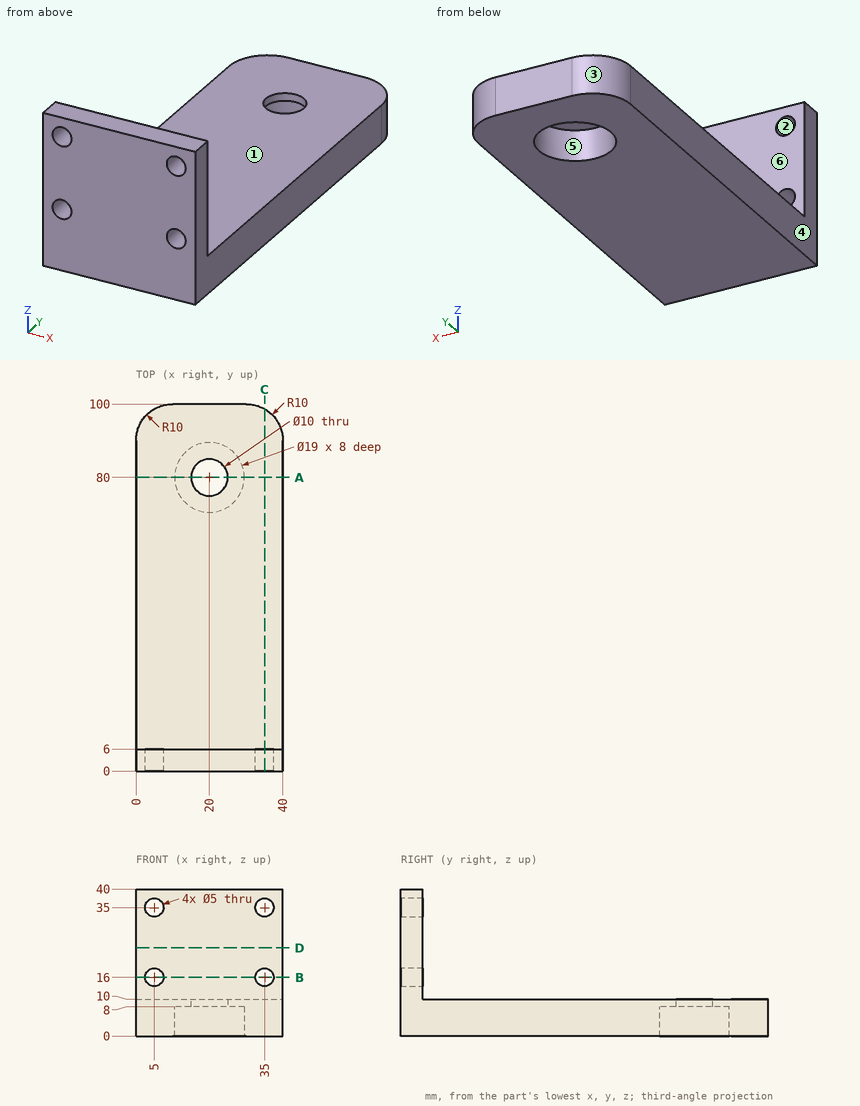
Answer from the drawing. Dimensions are ordinates in mm from the lowest x, y and z of the part. A direction names the side the tool comes from. Round coordinates to 2 decimals unless told otherwise and drop trailing zeros. Loops run counter-clockwise (first coordinate to the right, second up) from the corner with the lowest first, then second, coordinate; pieces in that order, holes last. Notation, with made-up numbers: (-5.75, -4) - (0.25, -4) arc R10 cw to (0.25, 9) - close; hole circle Ø2 at (19.5, 5.5). An arc over 180 degrees is marked (long way). Return JSON: item names as keys, results as strings. Group by question number.
1. Which of the six approach directions +Z, -Z, +X, -X, +Y, -Y give full straight-line access (tool end or side, diameter ignored) to the marked faces 4, 5 and 6?
2. The part is cut by section C-C on x = 35. Determine the outline of the cut face in (y, z).
3. The part is cut by section B-B on z = 16. Determine the outline of the cut face in (x, y), then the cut area to 3 significant figures.
4. The part is cut by section A-A on y = 80. Determine the outline of the cut face in (x, z), then the cut area to 3 significant figures.
5. The part is cut by section D-D on z = 24. Determine the outline of the cut face in (x, y).
6. Consider probe 1 along X at (y, z) = (4.05, 35); probe 2 along Y at (x, z) = (20, 9.55); probe 3 along Z at (x, y) = (11.5, 9.5). Determine where each line is inside the solid, lowest interval first.
7. Each of these flat-tipped pins is pushed along its axis until it touches: P1, Ø1, axis at x = 29, z = 21.5, coming from the +Y side; P2, Ø17, axis at x = 20, y = 80, coming from the +Z side; P3, Ø9, axis at x = 20, y = 80, coming from the +Z side. Where does it stop, or does it pass through?
8. The mould has two halves that part along Z. Classify the marked faces 1, 2 and 3: pulls with the +Z half, pulls with the -Z half, needs draft (parallel to the pull), parting line crosses it, or undercut.
Resolved:
{
 "1": {"face 4": "+Z, -Z, -X, +Y, -Y", "face 5": "-Z", "face 6": "+Z, +X, -X, +Y"},
 "2": {"outline": "(0, 0) - (98.66, 0) - (98.66, 10) - (6, 10) - (6, 13.5) - (0, 13.5) - close; (0, 18.5) - (6, 18.5) - (6, 32.5) - (0, 32.5) - close; (0, 37.5) - (6, 37.5) - (6, 40) - (0, 40) - close"},
 "3": {"outline": "(0, 0) - (2.5, 0) - (2.5, 6) - (0, 6) - close; (7.5, 0) - (32.5, 0) - (32.5, 6) - (7.5, 6) - close; (37.5, 0) - (40, 0) - (40, 6) - (37.5, 6) - close", "area": "180 mm²"},
 "4": {"outline": "(0, 0) - (10.5, 0) - (10.5, 8) - (15, 8) - (15, 10) - (0, 10) - close; (25, 8) - (29.5, 8) - (29.5, 0) - (40, 0) - (40, 10) - (25, 10) - close", "area": "228 mm²"},
 "5": {"outline": "(0, 0) - (40, 0) - (40, 6) - (0, 6) - close"},
 "6": {"probe 1": "x = 0 to 2.5, 7.5 to 32.5, 37.5 to 40", "probe 2": "y = 0 to 75, 85 to 100", "probe 3": "z = 0 to 10"},
 "7": {"P1": "stops at y = 6", "P2": "stops at z = 10", "P3": "passes through"},
 "8": {"face 1": "pulls with the +Z half", "face 2": "undercut", "face 3": "needs draft"}
}
